The model under review builds one solid part; all positions refer to its coordinate system, in mm. Face numbers are marked on the shaded views. Coordinates: 2 decimals unless noted, no trailing zeros. Write each loop counter-clockwise with the first axis right and the second up, starting at its lowest first coordinate (ties: lowest second). Pieces come first, ordered by that corner, then holes. Notation, with made-up numbers: M 5.25,28 L 46.25,28 A25 cw 46.25,62 Z; hole C 8,-8 d5. An arc over 180 degrees is marked long. Answer as a JSON object with one key per item and string values.
Autodesk Inventor part; units mm, degrees
ref_plane "YZ Plane" through (0, 0, 0) normal (1, 0, 0) x (0, 1, 0)
ref_plane "XZ Plane" through (0, 0, 0) normal (0, 1, 0) x (-1, 0, 0)
ref_plane "XY Plane" through (0, 0, 0) normal (0, 0, 1) x (1, 0, 0)
sketch "Sketch1" plane through (0, 0, 0) normal (0, 0, 1) x (1, 0, 0)
  circle A0 centre (0, 0) radius 30
extrude "Extrusion1" add sketch "Sketch1" along normal blind 10
sketch "Sketch2" plane through (0, 0, 0) normal (0, 0, 1) x (1, 0, 0)
  circle A0 centre (20, 0) radius 5
extrude "Extrusion2" cut sketch "Sketch2" along normal blind 10
pattern_circular "Circular Pattern1" count 6 over 360 about axis through (0, 0, -10) along (0, 0, 1) of "Extrusion2"
properties part number "22_pocket_circ"
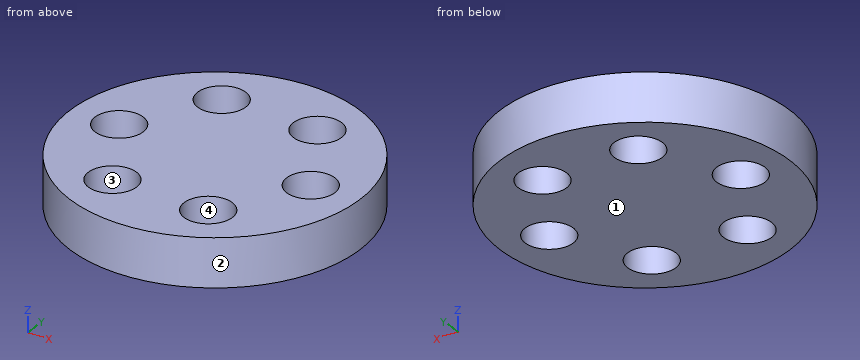
(1) Add section C-C on z = 4.75. Give the boundary of the cut face in (x, y).
Results list:
{"outline": "C 0,0 d60; hole C -20,0 d10; hole C -10,-17.32 d10; hole C -10,17.32 d10; hole C 10,-17.32 d10; hole C 10,17.32 d10; hole C 20,0 d10"}
(2) Wall thickness on line 1 along Y through (x, z) = (-10, 6); line 2 along X through (y, z) = (-14, 0.75); line 3 along X through (y, z) = (15, 3.75): over which ranges is each line inside the solid? List them lowest first. Write a range as from..to.
Results list:
{"line 1": "-28.28..-22.32, -12.32..12.32, 22.32..28.28", "line 2": "-26.53..-13.74, -6.26..6.26, 13.74..26.53", "line 3": "-25.98..-14.43, -5.57..5.57, 14.43..25.98"}
(3) Draft analysis for pull direction Y (two halves, no side actions). For the marked faces 1, 2, 3 and 4, state which applies: released by +Y, released by -Y, zero draft, split by the parting line, or undercut.
Results list:
{"face 1": "zero draft", "face 2": "split by the parting line", "face 3": "undercut", "face 4": "undercut"}
(4) Add section D-D on x = 20. Give the boundary of the cut face in (y, z).
Results list:
{"outline": "M -22.36,0 L -5,0 L -5,10 L -22.36,10 Z; M 5,0 L 22.36,0 L 22.36,10 L 5,10 Z"}
(5) For pin 1 Ø16 at (x, y) = (-10, 17.32) entering from +Z; pin 2 Ø4 at (x, z) = (23, 3.5) entering from +Y; pin 3 Ø1 at (x, z) = (23.5, 1.5) entering from +Y; pin 4 Ø4 at (x, z) = (20.5, 5) entering from -Y, all flat-tipped, find the tip position at first contact; note any pin that passes through.
Results list:
{"pin 1": "z = 10", "pin 2": "y = 21.42", "pin 3": "y = 19.26", "pin 4": "y = -23.62"}
(6) Add section B-B on y = 0. Give the boundary of the cut face in (x, z).
Results list:
{"outline": "M -30,0 L -25,0 L -25,10 L -30,10 Z; M -15,0 L 15,0 L 15,10 L -15,10 Z; M 25,0 L 30,0 L 30,10 L 25,10 Z"}
(7) Add section A-A on x = 8. Give the boundary of the cut face in (y, z).
Results list:
{"outline": "M -28.91,0 L -21.9,0 L -21.9,10 L -28.91,10 Z; M -12.74,0 L 12.74,0 L 12.74,10 L -12.74,10 Z; M 21.9,0 L 28.91,0 L 28.91,10 L 21.9,10 Z"}
